Geometry check sheet. Reference: the model listing, model coordinates, mm. A direction names the side the tool comes from. Round coordinates to 2 decimals unless told otherwise and drop trailing zeros. Loops run counter-clockwise (first coordinate to the right, second up) from the corner with the lowest first, then second, coordinate; pieces in that order, holes last. Notation, with made-up numbers: (57.5, 9) -> (112.5, 9) arc R25 cw to (112.5, 27) -> close; hole circle Ø6 at (45, -15.5). An arc over 180 degrees is marked (long way). Use a Markdown table: item, result. Add a question column.
Q1. Set-up check for faces 4 (the face through (-16, 5, -0.989)), 5 (the face through (14, 9.6, 13.98)): record each of +Z, -Z, +X, -X, +Y, -Y from which the full face is reachable in a straight line by a thin tool's end or side.
Q2. Sectioned sample at C-C, the plane y = 2. Enter the section's corners in (x, z), then the cut area to 3 significant figures.
Q3. Release check for a two-part mould opening along Z. For faces 1 (the face through (-16, 5, 1.217)), 2 (the face through (-16.7, 3.8, 4.017)), 3 (the face through (13.98, 9.6, -14)) record: released by +Z, released by -Z, zero draft, split by the parting line, or undercut.
Q4. Sectioned sample at B-B, the plane y = 7.5. Enter the section's corners in (x, z), then the cut area to 3 significant figures.
Q5. Gauge pin test, flat ends, axial feed: P1, Ø2.5, axis at x = -19.5, y = 6, coming from the -Z side; P2, Ø5, axis at y = 3.5, z = -7.5, coming from the -X side; P3, Ø5, axis at x = -18, y = 6.5, coming from the +Z side; P4, Ø12, axis at x = 9.5, z = -9, coming from the -Y side. Record the tip position at first contact, or that the pin passes through.
Q6. Material ranges on L1, parallel to Z at x = -18.5, y = 2.5; L2, parallel to X at y = 5, z = 2.3; L3, parallel to Z at x = -8, y = 1.75, recorded low to high.
Q7. Sectioned sample at A-A, the plane y = 5. Enter the section's corners in (x, z), then the cut area to 3 significant figures.
Autodesk Inventor part; units mm, degrees
ref_plane "YZ Plane" through (0, 0, 0) normal (1, 0, 0) x (0, 1, 0)
ref_plane "XZ Plane" through (0, 0, 0) normal (0, 1, 0) x (-1, 0, 0)
ref_plane "XY Plane" through (0, 0, 0) normal (0, 0, 1) x (1, 0, 0)
sketch "Эскиз1" plane through (0, 0, 0) normal (0, 1, 0) x (-1, 0, 0)
  arc A0 (9.8249, 1.217) -> (9.8505, -0.9889) centre (0, 0) ccw
  line L0 (-15.0002, 15) -> (-15.0002, -15)
  line L1 (-15.0002, 15) -> (0, 15)
  line L2 (-15.0002, -15) -> (0, -15)
  line L3 (9.8249, 1.217) -> (16.2051, 1.217)
  line L4 (13.6718, -0.9889) -> (9.8505, -0.9889)
  arc A1 (0, -15) -> (14.5136, -3.7889) centre (0, 0) ccw
  arc A2 (14.4521, 4.017) -> (0, 15) centre (0, 0) ccw
  line L5 (9.8505, -0.9889) -> (21.6521, -0.9889)
  line L6 (21.6521, -0.9889) -> (21.6521, -3.7889)
  line L7 (21.6521, -3.7889) -> (14.5136, -3.7889)
  line L8 (9.8249, 1.217) -> (21.6265, 1.217)
  line L9 (21.6265, 1.217) -> (21.6265, 4.017)
  line L10 (21.6265, 4.017) -> (14.4521, 4.017)
  point P0 (15, 0)
  dimension "d0" = 19.8
  dimension "d2" = 30
  dimension "d5" = 2.8
  dimension "d6" = 2.8
extrude "Выдавливание1" add sketch "Эскиз1" along normal blind 10
fillet "Сопряжение1" radius 4 4 edges at (-21.6265, 10, 2.617) (-21.6521, 10, -2.3889) (-21.6265, 0, 2.617) (-21.6521, 0, -2.3889)
sketch "Эскиз3" plane through (-14.4521, 0, 4.017) normal (0, 0, 1) x (1, 0, 0)
  arc A0 (-7.1744, 4) -> (-3.1744, 0) centre (-3.1744, 4) ccw
  line L0 (-3.1744, 0) -> (0, 0)
  line L1 (0, 0) -> (0, 10)
  line L2 (-3.1744, 10) -> (0, 10)
  arc A1 (-3.1744, 10) -> (-7.1744, 6) centre (-3.1744, 6) ccw
  line L3 (-7.1744, 4) -> (-7.1744, 6)
  line L4 (-7.1744, 5) -> (-3.6744, 5) construction
  point P0 (14.4521, 0)
  dimension "d20" = 3.5
hole "Отверстие2" at (-18.1265, 5, 4.017) direction (0, 0, -1) diameter 3 depth 8 tip angle 118
fillet "Сопряжение2" radius 2 2 edges at (15.0002, 5, 15) (15.0002, 5, -15)
chamfer "Фаска1" distance 1 angle 45 16 edges at (9.8993, 10, -0.1148) (9.8993, 0, -0.1148) (6.5001, 10, 15) (14.4144, 10, 14.4142) (15.0002, 10, 0) (14.4144, 10, -14.4142) (6.5001, 10, -15) (-9.1697, 10, -11.8708) (-9.0759, 10, 11.9427) (6.5001, 0, 15) (14.4144, 0, 14.4142) (15.0002, 0, 0) (14.4144, 0, -14.4142) (6.5001, 0, -15) (-9.1697, 0, -11.8708) (-9.0759, 0, 11.9427)
properties part number "BasicMount 19.5mm"
Values:
| question | item | result |
|---|---|---|
| 1 | face 4 | -X, +Y, -Y |
| 1 | face 5 | +Z, +X, +Y |
| 2 | outline | (-21.12, -3.79) -> (-14.51, -3.79) arc R15 ccw to (0, -15) -> (13, -15) arc R2 ccw to (15, -13) -> (15, 13) arc R2 ccw to (13, 15) -> (0, 15) arc R15 ccw to (-14.45, 4.02) -> (-21.09, 4.02) -> (-21.09, 1.22) -> (-9.82, 1.22) arc R9.9 cw (long way) to (-9.85, -0.99) -> (-21.12, -0.99) -> close |
| 2 | area | 518 mm^2 |
| 3 | face 1 | undercut |
| 3 | face 2 | released by +Z |
| 3 | face 3 | released by -Z |
| 4 | outline | (-21.36, -3.79) -> (-14.51, -3.79) arc R15 ccw to (0, -15) -> (13, -15) arc R2 ccw to (15, -13) -> (15, 13) arc R2 ccw to (13, 15) -> (0, 15) arc R15 ccw to (-14.45, 4.02) -> (-21.33, 4.02) -> (-21.33, 1.22) -> (-9.82, 1.22) arc R9.9 cw (long way) to (-9.85, -0.99) -> (-21.36, -0.99) -> close |
| 4 | area | 519 mm^2 |
| 5 | P1 | z = -3.79 |
| 5 | P2 | x = -14.14 |
| 5 | P3 | z = 4.02 |
| 5 | P4 | y = 0 |
| 6 | L1 | -3.79 to -0.99, 1.22 to 4.02 |
| 6 | L2 | -21.63 to -19.63, -16.63 to -9.63, 9.63 to 15 |
| 6 | L3 | -12.69 to -5.83, 5.83 to 12.69 |
| 7 | outline | (-21.65, -3.79) -> (-19.63, -3.79) -> (-19.63, -0.99) -> (-21.65, -0.99) -> close; (-21.63, 1.22) -> (-19.63, 1.22) -> (-19.63, 4.02) -> (-21.63, 4.02) -> close; (-16.63, -3.79) -> (-14.51, -3.79) arc R15 ccw to (0, -15) -> (13, -15) arc R2 ccw to (15, -13) -> (15, 13) arc R2 ccw to (13, 15) -> (0, 15) arc R15 ccw to (-14.45, 4.02) -> (-16.63, 4.02) -> (-16.63, 1.22) -> (-9.82, 1.22) arc R9.9 cw (long way) to (-9.85, -0.99) -> (-16.63, -0.99) -> close |
| 7 | area | 504 mm^2 |
